Verification items for the finished model (mm, model axes). Face numbers are marked on the shaded views. A direction names the side the tool comes from. Give positions to 0.01 mm unless a question says otherwise; leave off trailing zeros. Order: outer loops, then holes, each group sorted by start corner. A loop starts at its lowest first (then second) coordinate and runs counter-clockwise, first axis right, second up. Notation, with made-up numbers: (-36, -7.5) - (10, -7.5) arc R5 cw to (10, -2.5) - close; hole circle Ø4 at (45, 10). An arc over 180 degrees is marked (long way). Answer as a JSON object with one key per item and string values.
```python
from build123d import *

# Parameters (mm, degrees)
F1_DEPTH = 25
F4_D     = 5.1054
F4_DEPTH = 25
F4_TIP   = 1.5338169022
F5_D     = 6.7564
F5_DEPTH = 25
F5_TIP   = 2.0298273432


with BuildPart() as f1:
    # F0 (on Top) → F1 (new body)
    with BuildSketch(Plane.XY):
        with BuildLine():
            ThreePointArc((45, 0), (0, -45), (-45, 0))
            Line((-45, 0), (-68, 0))
            Line((-68, 0), (-68, -4.880737979))
            Line((-68, -4.880737979), (-52.2726352577, -4.880737979))
            ThreePointArc((-52.2726352577, -4.880737979), (-5.3689869527, -52.2247448926), (50.1862195886, -15.4140638188))
            Line((50.1862195886, -15.4140638188), (68, -15.4140638188))
            Line((68, -15.4140638188), (68, 0))
            Line((68, 0), (45, 0))
        make_face()
    extrude(amount=F1_DEPTH)

    # F4
    with Locations(Plane(origin=(0, 0, 0), x_dir=(-1, 0, 0), z_dir=(0, 1, 0))):
        with Locations((-60, 6), (-60, 19)):
            Hole(F4_D / 2, depth=F4_DEPTH)
            with Locations((0, 0, -(F4_DEPTH + F4_TIP / 2))):  # 118° drill point
                Cone(0, F4_D / 2, F4_TIP, mode=Mode.SUBTRACT)

    # F5
    with Locations(Plane(origin=(0, 0, 0), x_dir=(-1, 0, 0), z_dir=(0, 1, 0))):
        with Locations((60, 6), (60, 19)):
            Hole(F5_D / 2, depth=F5_DEPTH)
            with Locations((0, 0, -(F5_DEPTH + F5_TIP / 2))):  # 118° drill point
                Cone(0, F5_D / 2, F5_TIP, mode=Mode.SUBTRACT)


solid = f1.part
```
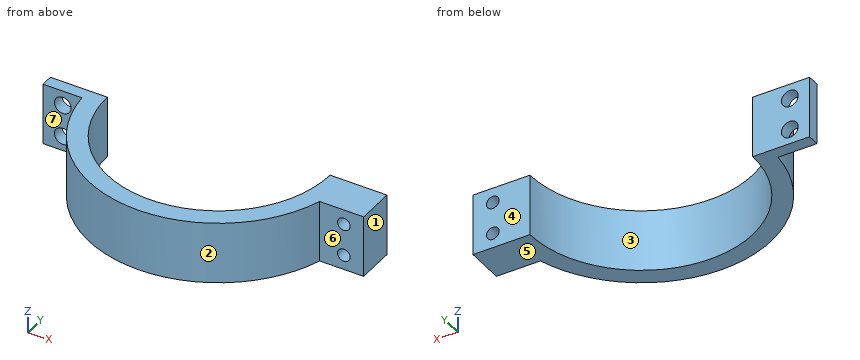
(1) Section check C-C (x = 0). Record the cut outline in (y, z).
Computed values:
{"outline": "(-52.5, 0) - (-45, 0) - (-45, 25) - (-52.5, 25) - close"}
(2) Section check B-B (y = -31.5). Record the cut outline in (x, z).
Computed values:
{"outline": "(-42, 0) - (-32.14, 0) - (-32.14, 25) - (-42, 25) - close; (32.14, 0) - (42, 0) - (42, 25) - (32.14, 25) - close"}
(3) Gauge pin test, flat ends, axial feed: pin 1 Ø6 at (x, z) = (-17, 20) entering from -Y; pin 2 Ø4.5 at (x, z) = (-57, 11.5) entering from -Y; pin 3 Ø5 at (y, z) = (-45.5, 18) entering from -X; pin 4 Ø3 at (x, z) = (60, 19) entering from +Y. Record the tip position at first contact, or that the pin passes through.
Computed values:
{"pin 1": "stops at y = -50.6", "pin 2": "stops at y = -4.88", "pin 3": "stops at x = -30.12", "pin 4": "passes through"}
(4) Section check A-A (z = 19). Record the cut outline in (x, y).
Computed values:
{"outline": "(-68, -4.88) - (-63.38, -4.88) - (-63.38, 0) - (-68, 0) - close; (-56.62, -4.88) - (-52.27, -4.88) arc R52.5 ccw to (50.19, -15.41) - (57.45, -15.41) - (57.45, 0) - (45, 0) arc R45 cw to (-45, 0) - (-56.62, 0) - close; (62.55, -15.41) - (68, -15.41) - (68, 0) - (62.55, 0) - close"}
(5) Section check D-D (y = -26). Record the cut outline in (x, z).
Computed values:
{"outline": "(-45.61, 0) - (-36.73, 0) - (-36.73, 25) - (-45.61, 25) - close; (36.73, 0) - (45.61, 0) - (45.61, 25) - (36.73, 25) - close"}
(6) Access from +Z, -Z, +X, -X, +Y, -Y to the whole of each face (thin tool, end or side, straight path). Record for the marked faces 5, 6 and 7.
Computed values:
{"face 5": "-Z, +X, -X, +Y, -Y", "face 6": "+Z, -Z, +X, -Y", "face 7": "+Z, -Z, -X, -Y"}
(7) Release check for a two-part mould opening along X. For the marked faces 1, 2, 3 and 4 record: pulls with the +X half, pulls with the -X half, needs draft (parallel to the pull), parting line crosses it, or undercut.
Computed values:
{"face 1": "pulls with the +X half", "face 2": "parting line crosses it", "face 3": "undercut", "face 4": "needs draft"}
(8) Material ranges on line 1 along Z through (x, y) = (-60, -2.35); line 2 along Z through (x, y) = (60, -11.75); line 3 along Y through (x, z) = (-55, 18), recorded low to high. Write a range as [from, to].
Computed values:
{"line 1": "z = [0, 2.62], [9.38, 15.62], [22.38, 25]", "line 2": "z = [0, 3.45], [8.55, 16.45], [21.55, 25]", "line 3": "y = [-4.88, 0]"}
